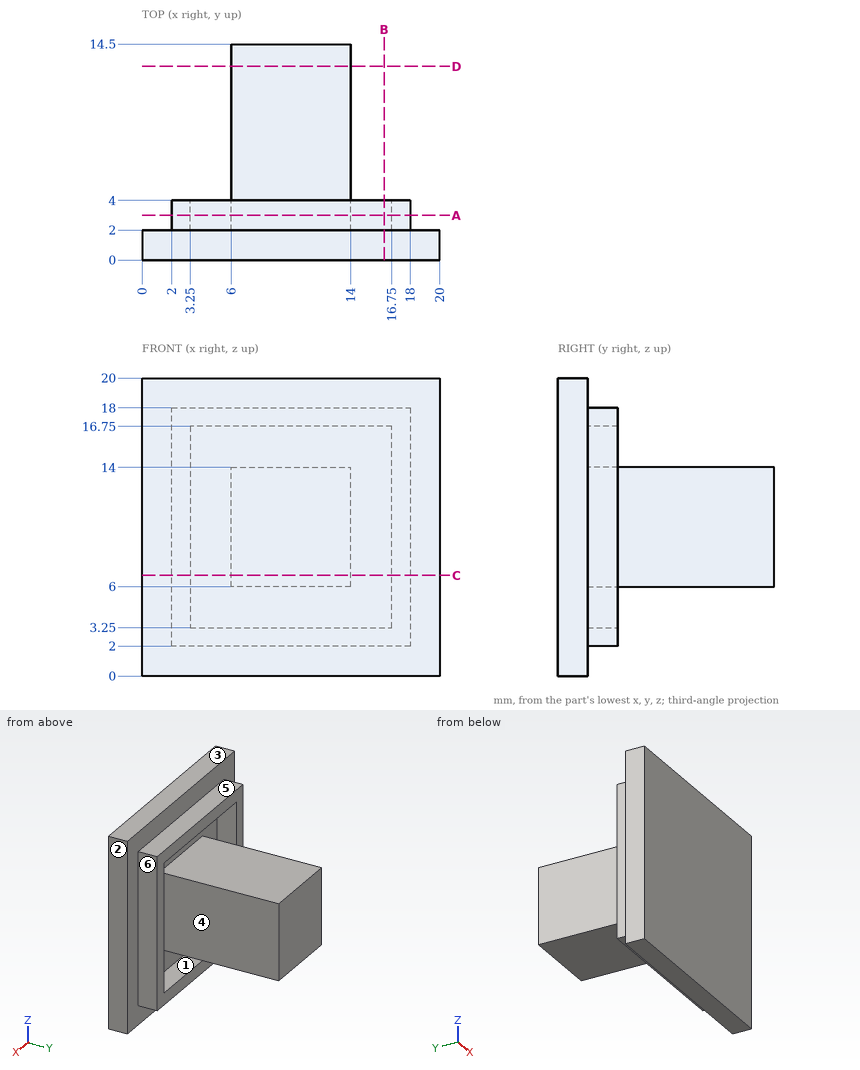
Study the drawing (mm; zero at the part's minimum x, y, z) and answer. A direction names the side the tool comes from. Round coordinates to 2 decimals unless told otherwise and drop trailing zeros. Write each loop counter-clockwise with the first axis right and the second up, starting at its lowest first coordinate (ties: lowest second). Pieces come first, ordered by that corner, then holes.
Q1. Find section B-B on x = 16.25. Determine the outline of the cut face in (y, z).
Values:
outline: (0, 0) - (2, 0) - (2, 2) - (4, 2) - (4, 3.25) - (2, 3.25) - (2, 16.75) - (4, 16.75) - (4, 18) - (2, 18) - (2, 20) - (0, 20) - close
Q2. Find section C-C on z = 6.75. Determine the outline of the cut face in (x, y).
Values:
outline: (0, 0) - (20, 0) - (20, 2) - (18, 2) - (18, 4) - (16.75, 4) - (16.75, 2) - (14, 2) - (14, 14.5) - (6, 14.5) - (6, 2) - (3.25, 2) - (3.25, 4) - (2, 4) - (2, 2) - (0, 2) - close
Q3. Straight lines are drawn through the part: line 1 (X direction, y = 3.5, z = 11); line 2 (Z direction, x = 7, y = 5.75); line 3 (Y direction, x = 1, z = 4). For each, find the intervals that lie inside material, in ascending order.
Values:
line 1: x = 2 to 3.25, 6 to 14, 16.75 to 18
line 2: z = 6 to 14
line 3: y = 0 to 2
Q4. Find section D-D on y = 13. Determine the outline of the cut face in (x, z), and give its area (3 significant figures).
Values:
outline: (6, 6) - (14, 6) - (14, 14) - (6, 14) - close
area: 64.0 mm2
Q5. The mould has two halves that part along Z. Classify the marked faces 1, 2 and 3: released by +Z, released by -Z, zero draft, split by the parting line, or undercut.
Values:
face 1: undercut
face 2: zero draft
face 3: released by +Z
Q6. Flat-ended cylindrical pins translate along their axes: P1, Ø0.6, axis at x = 12.5, y = 3, coming from the +Z side; P2, Ø8, axis at y = 12, z = 12.5, coming from the -X side; P3, Ø2, axis at x = 12.5, y = 6.5, coming from the +Z side. Find the tip coordinate at first contact, or state that the pin passes through.
Values:
P1: stops at z = 18
P2: stops at x = 6
P3: stops at z = 14
Q7. A tool of negligible diameter and unlimited length cuts with its end or side. For the marked faces 4, 5 and 6, from which of +Z, -Z, +X, -X, +Y, -Y can it reach the whole face along a straight path? Write none if from no direction.
Values:
face 4: +Y
face 5: +Z, +X, -X, +Y
face 6: +Z, -Z, +X, +Y
Q8. Find section A-A on y = 3. Determine the outline of the cut face in (x, z), and give its area (3 significant figures).
Values:
outline: (2, 2) - (18, 2) - (18, 18) - (2, 18) - close; (6, 6) - (14, 6) - (14, 14) - (6, 14) - close; hole (3.25, 3.25) - (16.75, 3.25) - (16.75, 16.75) - (3.25, 16.75) - close
area: 138 mm2
